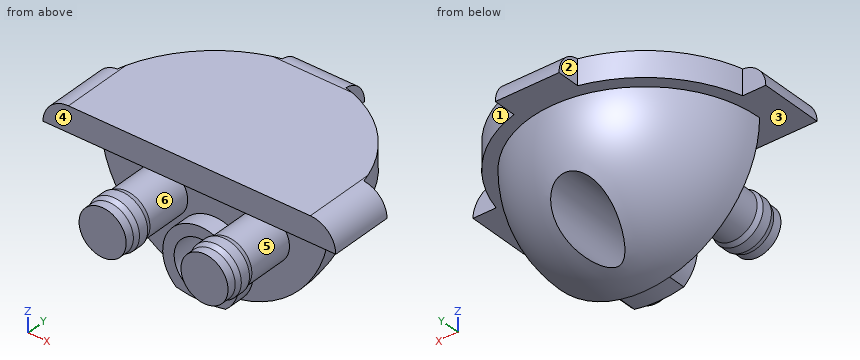
```python
from build123d import *

# Parameters (mm, degrees)
SKETCH_1_R               = 10
EXTRUDE_1_DEPTH          = 2
REVOLVE_1_ANGLE          = 180
SKETCH_5_R               = 2.1
CUT_EXTRUDE_1_DEPTH      = 10
SKETCH_6_R               = 1.85
EXTRUDE_2_DEPTH          = 6
EXTRUDE_START            = 1.38
SKETCH_7_R               = 2.1
EXTRUDE_3_DEPTH          = 1.38
SKETCH_10_W              = 5
SKETCH_10_H              = 23
EXTRUDE_4_DEPTH          = 2
PATTERN_CIRCULAR_3_COUNT = 4
FILLET_3_R               = 2
SKETCH_11_W              = 19.364916732
SKETCH_11_H              = 12.045075347
CUT_EXTRUDE_2_DEPTH      = 10


with BuildPart() as part:
    # 草图1 → 凸台-拉伸1 (new body)
    with BuildSketch(Plane.XY):
        Circle(SKETCH_1_R)
    extrude(amount=EXTRUDE_1_DEPTH)

    # 草图2 → 旋转1 (revolve)
    with BuildSketch(Plane(origin=(0, 0, 0), x_dir=(-1, 0, 0), z_dir=(0, 0, -1))):
        with BuildLine():
            Line((0, 9), (0, 0))
            Line((0, 0), (9, 0))
            ThreePointArc((9, 0), (6.363961031, 6.363961031), (0, 9))
        make_face()
    revolve(axis=Axis((0, 0, 0), (0, -1, 0)), revolution_arc=REVOLVE_1_ANGLE)

    # 草图5 → 切除-拉伸1 (cut)
    with BuildSketch(Plane.XZ):
        with Locations(Location((0, -6.5, 0), (0, 0, 270))):
            Circle(SKETCH_5_R)
    extrude(amount=-CUT_EXTRUDE_1_DEPTH, mode=Mode.SUBTRACT)

    # 草图6 → 凸台-拉伸2 (add)
    with BuildSketch(Plane.XZ):
        with Locations(Location((-4, -3.177350455, 0), (0, 0, 90))):
            Circle(SKETCH_6_R)
    extrude_2 = extrude(amount=EXTRUDE_2_DEPTH)

    # 镜向1: 凸台-拉伸2 across plane
    add(extrude_2.mirror(Plane(origin=(0, 0, 0), x_dir=(0, 0, 1), z_dir=(1, 0, 0))))

    # 草图7 → 凸台-拉伸3 (add)
    with BuildSketch(Plane.XZ.offset(EXTRUDE_START)):
        with BuildLine():
            ThreePointArc((1.939830866, -8.788461538), (0, -3.5), (-1.939830866, -8.788461538))
            ThreePointArc((-1.939830866, -8.788461538), (0, -9), (1.939830866, -8.788461538))
        make_face()
        with Locations(Location((0, -6.5, 0), (0, 0, 270))):
            Circle(SKETCH_7_R, mode=Mode.SUBTRACT)
    extrude(amount=-EXTRUDE_3_DEPTH)

    # 草图8 → 旋转2 (revolve)
    with BuildSketch(Plane.XY.offset(-3.177350455), mode=Mode.PRIVATE) as revolve_2_sk:
        Polygon((4, -3.675756774), (2.15, -3.675756774), (2, -4.087878387), (2, -4.887878387), (2.15, -5.3), (4, -5.3), align=None)
    revolve_2 = revolve(revolve_2_sk.sketch.rotate(Axis((4, -5.3, -3.177350455), (0, 1, 0)), 270), axis=Axis((4, -5.3, -3.177350455), (0, 1, 0)))

    # 镜向2: 旋转2 across plane
    add(revolve_2.mirror(Plane(origin=(0, 0, 0), x_dir=(0, 0, 1), z_dir=(1, 0, 0))))

    # 草图10 → 凸台-拉伸4 (add)
    with BuildSketch(Plane.XY.offset(2)):
        Rectangle(SKETCH_10_W, SKETCH_10_H)
    extrude_4 = extrude(amount=-EXTRUDE_4_DEPTH)

    # 阵列(圆周)3: 凸台-拉伸4 ×4 about axis
    pattern_circular_3_axis = Axis((0, 0, 0), (0, 0, 1))
    for i in range(1, PATTERN_CIRCULAR_3_COUNT):
        add(extrude_4.rotate(pattern_circular_3_axis, i * 360 / PATTERN_CIRCULAR_3_COUNT))

    # 圆角3
    fillet_3_edges = [part.edges().sort_by_distance(p)[0] for p in [
        (0, 11.5, 2),
        (0, -11.5, 2),
        (11.5, 0, 2),
        (-11.5, 0, 2),
    ]]
    fillet(fillet_3_edges, radius=FILLET_3_R - 0.0001)  # a hair under: the kernel refuses the full size

    # 草图11 → 切除-拉伸2 (cut)
    with BuildSketch(Plane(origin=(0, 0, 0), x_dir=(-1, 0, 0), z_dir=(0, 0, -1))):
        with Locations((0, -8.522537674)):
            Rectangle(SKETCH_11_W, SKETCH_11_H)
    extrude(amount=-CUT_EXTRUDE_2_DEPTH, mode=Mode.SUBTRACT)


solid = part.part
```
CAD build for the part. Positions are in the model's coordinates, mm. Face numbers are marked on the shaded views. A direction names the side the tool comes from. Round coordinates to 2 decimals unless told otherwise and drop trailing zeros. Order: outer loops, then holes, each group sorted by start corner. A loop starts at its lowest first (then second) coordinate and runs counter-clockwise, first axis right, second up.
Item 1: Probe line 1 along X through (y, z) = (-0.5, -4); line 2 along Z through (x, y) = (0, 6.25); line 3 along Z through (x, y) = (-3.75, -0.25). List the from-to ranges inside material, lowest first.
Item 2: Saw through at B-B on z = -6.5. Write the cut outline in (x, y).
Item 3: Pin check, flat tips, straight feed: pin 1 (7 mm diameter, centred on x = -5, y = 7, fed in from -Z); pin 2 (1.5 mm diameter, centred on x = -1, y = 0.5, fed in from -Z); pin 3 (0.5 mm diameter, centred on x = 10.5, z = 1, fed in from +Y). Stop position of each tip, or through.
Item 4: Saw through at A-A on y = -2.25. State how many separate pieces and enclosed holes the cut face has, then the cut area to 3 significant figures.
Item 5: Saw through at D-D on x = -7. Write the cut outline in (y, z).
Item 6: Tool access for the marked faces 1 and 2: list every direction of +Z, -Z, +X, -X, +Y, -Y with a clear straight run to the whole face (end or side of a thin tool).
Item 7: Mould opens along Y. For the marked faces 3, 4, 5 and 6 say: pulls with the +Y half, pulls with the -Y half, needs draft (parallel to the pull), parting line crosses it, or undercut.
Reported:
1. line 1: x = -5.66 to -2.34, -1.66 to 1.66, 2.34 to 5.66
1. line 2: z = -4.4 to 2
1. line 3: z = -5.01 to -1.34, 0 to 2
2. outline: (-6.22, 0) - (-3, 0) - (-3, -1.38) - (-2.1, -1.38) - (-2.1, 5.86) arc R6.22 ccw to start; (2.1, -1.38) - (3, -1.38) - (3, 0) - (6.22, 0) arc R6.22 ccw to (2.1, 5.86) - close
3. pin 1: stops at z = -7.41
3. pin 2: stops at z = -8.99
3. pin 3: stops at y = 2.5
4. separate pieces: 3
4. enclosed holes: 0
4. area: 65.8 mm2
5. outline: (-2.5, 0) - (0, 0) - (0, -5.66) arc R5.66 ccw to (5.66, 0) - (7.14, 0) - (7.14, 2) - (-2.5, 2) - close
6. face 1: +Z, -Z, +X, +Y
6. face 2: +Z, -Z, -X, +Y
7. face 3: needs draft
7. face 4: pulls with the -Y half
7. face 5: undercut
7. face 6: undercut
